Geometry: final body of the model. Coordinates: model frame, mm. Give positions to 0.01 mm unless a question says otherwise; leave off trailing zeros. Order: outer loops, then holes, each group sorted by start corner. A loop starts at its lowest first (then second) coordinate and runs counter-clockwise, first axis right, second up. Notation, with made-up numbers: (64, 35) - (71, 35) arc R9 cw to (71, 41) - close; hole circle Ø4 at (-7.5, 12.25). An arc over 180 degrees is marked (long way). One line per item, written item: value.
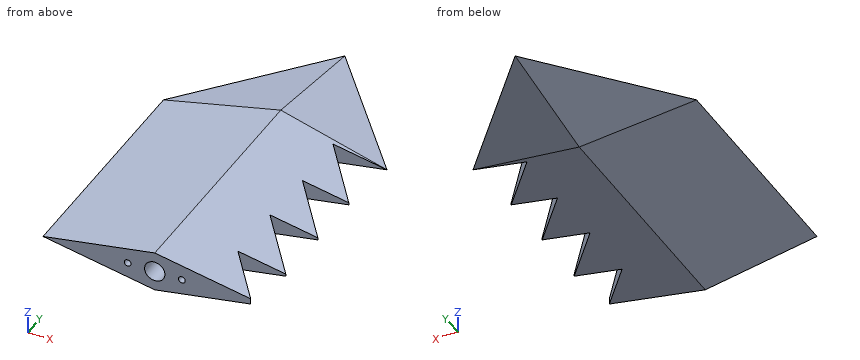
```python
from build123d import *

# Parameters (mm, degrees)
BOSS_EXTRUDE1_DEPTH      = 9.525
BOSS_EXTRUDE1_DEPTH_BACK = 9.525
CUT_EXTRUDE1_DEPTH       = 373.680910299
CUT_EXTRUDE2_DEPTH       = 373.680910299
SKETCH5_W                = 97.518379051
SKETCH5_H                = 136.419580789
CUT_EXTRUDE3_DEPTH       = 739.741184154
SKETCH6_W                = 75.100700845
SKETCH6_H                = 154.277977479
CUT_EXTRUDE4_DEPTH       = 748.678846608
SKETCH7_R                = 4.7625
CUT_EXTRUDE5_DEPTH       = 254
CUT_EXTRUDE6_DEPTH       = 752.699804454
CUT_EXTRUDE6_DEPTH_BACK  = 752.699804454
SKETCH8_W                = 222.997610285
SKETCH8_H                = 218.448411489
SKETCH11_R               = 1.5875
CUT_EXTRUDE9_DEPTH       = 12.7


with BuildPart() as part:
    # Sketch1 → Boss-Extrude1 (new, two sides: drawn at the far end of the back side and taken through both)
    with BuildSketch(Plane.XY.offset(-BOSS_EXTRUDE1_DEPTH_BACK)):
        Polygon((101.792411443, 735.656458749), (49.404911443, 673.557276224), (49.404911443, 396.497366015), (154.179911443, 396.497366015), (154.179911443, 556.636391043), (128.683999881, 589.063224066), (151.148766449, 589.063224066), (128.683999881, 617.634912224), (151.148766449, 617.634912224), (129.452026088, 645.229790529), (151.148766449, 645.229790529), (128.876006433, 673.557276224), (154.179911443, 673.557276224), align=None)
    extrude(amount=BOSS_EXTRUDE1_DEPTH + BOSS_EXTRUDE1_DEPTH_BACK)

    # Sketch2 → Cut-Extrude1 (cut, through all)
    with BuildSketch(Plane(origin=(0, 396.497366015, 0), x_dir=(-1, 0, 0), z_dir=(0, -1, 0))):
        Polygon((-49.404911443, 0), (-101.792411443, -9.525), (-154.179911443, 0), (-159.65732669, 0), (-159.65732669, -13.649148588), (-44.158493861, -13.649148588), (-44.158493861, 0), align=None)
    extrude(amount=-CUT_EXTRUDE1_DEPTH, mode=Mode.SUBTRACT)

    # Sketch3 → Cut-Extrude2 (cut, through all)
    with BuildSketch(Plane.XZ.offset(-396.497366015)):
        Polygon((49.404911443, 0), (101.792411443, -9.525), (154.179911443, 0), (159.580570647, 0), (159.580570647, -14.500746269), (43.682013433, -14.500746269), (43.682013433, 0), align=None)
    extrude(amount=-CUT_EXTRUDE2_DEPTH, mode=Mode.SUBTRACT)

    # Sketch5 → Cut-Extrude3 (cut, through all)
    with BuildSketch(Plane(origin=(26.430459561, 22.297003663, 133.782021979), x_dir=(0.9815360247212257, -0.031445805879602766, -0.1886748352776165), z_dir=(0.1912773697394791, 0.16136352846789567, 0.9681811708073739))):
        with Locations((89.248369642, 700.742830845)):
            Rectangle(SKETCH5_W, SKETCH5_H)
    cut_extrude3 = extrude(amount=CUT_EXTRUDE3_DEPTH, mode=Mode.SUBTRACT)

    # Sketch6 → Cut-Extrude4 (cut, through all)
    with BuildSketch(Plane(origin=(-18.981895096, 16.01331916, 96.079914958), x_dir=(0.9815360247212258, 0.03144580587960229, 0.18867483527761636), z_dir=(-0.19127736973947887, 0.1613635284678934, 0.9681811708073744))):
        with Locations((98.873573013, 697.792784398)):
            Rectangle(SKETCH6_W, SKETCH6_H)
    cut_extrude4 = extrude(amount=CUT_EXTRUDE4_DEPTH, mode=Mode.SUBTRACT)

    # Mirror1: Cut-Extrude3, Cut-Extrude4 across plane
    add(cut_extrude3.mirror(Plane.XY), mode=Mode.SUBTRACT)
    add(cut_extrude4.mirror(Plane.XY), mode=Mode.SUBTRACT)

    # Sketch7 → Cut-Extrude5 (cut)
    with BuildSketch(Plane.XZ.offset(-396.497366015)):
        with Locations(Location((101.792411443, 0, 0), (0, 0, 270))):
            Circle(SKETCH7_R)
    extrude(amount=-CUT_EXTRUDE5_DEPTH, mode=Mode.SUBTRACT)

    # Sketch8 → Cut-Extrude6 (cut, two sides: drawn at the far end of the back side and taken through both)
    with BuildSketch(Plane.XY.offset(-CUT_EXTRUDE6_DEPTH_BACK)):
        with Locations((89.854155539, 456.852706638)):
            Rectangle(SKETCH8_W, SKETCH8_H)
    extrude(amount=CUT_EXTRUDE6_DEPTH + CUT_EXTRUDE6_DEPTH_BACK, mode=Mode.SUBTRACT)

    # Sketch11 → Cut-Extrude9 (cut)
    with BuildSketch(Plane.XZ.offset(-566.076912382)):
        with Locations(Location((89.092411443, 0, 0), (0, 0, 270))):
            Circle(SKETCH11_R)
        with Locations(Location((114.492411443, 0, 0), (0, 0, 270))):
            Circle(SKETCH11_R)
    extrude(amount=-CUT_EXTRUDE9_DEPTH, mode=Mode.SUBTRACT)


solid = part.part
```
1) Section B-B, the plane z = -7. Return loops of the section in (x, y), then the cut area to 3 significant figures.
Answers below:
outline: (87.9, 566.08) - (115.68, 566.08) - (115.68, 677.19) - (101.79, 693.66) - (87.9, 677.19) - close
area: 3,310 mm^2
2) Section C-C, the plane x = 62. Return loops of the section in (y, z).
Answers below:
outline: (566.08, -2.29) - (674.75, -2.29) - (688.49, 0) - (674.75, 2.29) - (566.08, 2.29) - close
3) Section A-A, the plane y = 586. Return loops of the section in (x, z) (1 decimal), then the cut area to 3 significant figures.
Answers below:
outline: (49.4, 0) - (101.8, -9.5) - (131.1, -4.2) - (131.1, 4.2) - (101.8, 9.5) - close; hole circle Ø9.5 at (101.8, 0)
area: 830 mm^2
4) First-contact query: pin 1 (5 mm diameter, centred on x = 111, y = 700, fed in from +Z); pin 2 (1.9 mm diameter, centred on x = 114.49, z = 0, fed in from +Y); pin 3 (1 mm diameter, centred on x = 133, y = 647, fed in from +Z). Flat tips, straight axial feed; report the tip coordinate or a pass-through.
Answers below:
pin 1: z = 4.77
pin 2: y = 721.73
pin 3: z = 3.94
5) Material intervals for line 1 along Z through (x, y) = (98, 622); line 2 along Z through (x, y) = (109, 712); line 3 along Z through (x, y) = (118, 582), sorted ascending.
Answers below:
line 1: -8.84 to -2.88, 2.88 to 8.84
line 2: -2.52 to 2.52
line 3: -6.58 to 6.58
6) Section D-D, the plane y = 612. Return loops of the section in (x, z) (1 decimal), then the cut area to 3 significant figures.
Answers below:
outline: (49.4, 0) - (101.8, -9.5) - (133.1, -3.8) - (133.1, 3.8) - (101.8, 9.5) - close; hole circle Ø9.5 at (101.8, 0)
area: 846 mm^2
